Source: CAD feature listing. Evaluate the final solid. Frame: model axes, mm. A direction names the side the tool comes from. Give positions to 0.01 mm unless a question says otherwise; leave off trailing zeros. Order: outer loops, then holes, each group sorted by start corner. A loop starts at its lowest first (then second) coordinate and runs counter-clockwise, first axis right, second up.
from build123d import *

# Parameters (mm, degrees)
SKETCH1_R           = 6
BOSS_EXTRUDE1_DEPTH = 2
SKETCH2_R           = 3.5
SKETCH2_R_2         = 2.5
BOSS_EXTRUDE2_DEPTH = 3
SKETCH3_R           = 0.75
CUT_EXTRUDE1_DEPTH  = 2.5
CHAMFER1_SIZE       = 0.5
SKETCH5_R           = 1.25
CUT_EXTRUDE3_DEPTH  = 10.848857924


with BuildPart() as part:
    # Sketch1 → Boss-Extrude1 (new body)
    with BuildSketch(Plane.XY):
        Circle(SKETCH1_R)
    extrude(amount=BOSS_EXTRUDE1_DEPTH)

    # Sketch2 → Boss-Extrude2 (add)
    with BuildSketch(Plane(origin=(0, 0, 0), x_dir=(-1, 0, 0), z_dir=(0, 0, -1))):
        with Locations(Location((0, 0, 0), (0, 0, 180))):
            Circle(SKETCH2_R)
        Circle(SKETCH2_R_2, mode=Mode.SUBTRACT)
    extrude(amount=BOSS_EXTRUDE2_DEPTH)

    # Sketch3 → Cut-Extrude1 (cut)
    with BuildSketch(Plane.XY.offset(2)):
        with Locations((0, 5)):
            Circle(SKETCH3_R)
        with Locations((5.001, 0.001)):
            Circle(SKETCH3_R)
        with Locations((0.002, -5)):
            Circle(SKETCH3_R)
        with Locations((-4.999, -0.001)):
            Circle(SKETCH3_R)
    extrude(amount=-CUT_EXTRUDE1_DEPTH, mode=Mode.SUBTRACT)

    # Chamfer1
    # the kernel refuses this chamfer: 0.5 mm, written as the material it takes off along each edge
    with BuildSketch(Plane(origin=(0, 0, 0), x_dir=(1, 0, 0), z_dir=(0, -1, 0))) as chamfer1_piece_1:
        Polygon((6, CHAMFER1_SIZE), (6 - CHAMFER1_SIZE, 0), (6, 0), align=None)
    revolve(axis=Axis((0, 0, 0), (0, 0, 1)), mode=Mode.SUBTRACT)
    with BuildSketch(Plane(origin=(0, 0, 2), x_dir=(1, 0, 0), z_dir=(0, -1, 0))) as chamfer1_piece_2:
        Polygon((6, -CHAMFER1_SIZE), (6 - CHAMFER1_SIZE, 0), (6, 0), align=None)
    revolve(axis=Axis((0, 0, 2), (0, 0, 1)), mode=Mode.SUBTRACT)
    with BuildSketch(Plane(origin=(0, 0, -3), x_dir=(1, 0, 0), z_dir=(0, 1, 0))) as chamfer1_piece_3:
        Polygon((3.5, -CHAMFER1_SIZE), (3.5 - CHAMFER1_SIZE, 0), (3.5, 0), align=None)
    revolve(axis=Axis((0, 0, -3), (0, 0, -1)), mode=Mode.SUBTRACT)

    # Sketch5 → Cut-Extrude3 (cut, through all)
    with BuildSketch(Plane.XY.offset(2)):
        Circle(SKETCH5_R)
    extrude(amount=-CUT_EXTRUDE3_DEPTH, mode=Mode.SUBTRACT)


solid = part.part
1) Section query A-A on z = -0.75. Output: boundary loops of the cut face in (x, y), and give its area (3 significant figures).
Checks:
outline: circle Ø7 at (0, 0); hole circle Ø5 at (0, 0)
area: 18.8 mm2
2) Section query B-B on z = 1.05. Output: boundary loops of the cut face in (x, y), and give its area (3 significant figures).
Checks:
outline: circle Ø12 at (0, 0); hole circle Ø1.5 at (-5, 0); hole circle Ø2.5 at (0, 0); hole circle Ø1.5 at (0, -5); hole circle Ø1.5 at (0, 5); hole circle Ø1.5 at (5, 0)
area: 101 mm2
3) Ray query, L1, parallel to Y at x = 0, z = 1; L2, parallel to Y at x = -1.75, z = -2; L3, parallel to X at y = -2.25, z = -2.45. Return the intervals inside material, ascending.
Checks:
L1: y = -6 to -5.75, -4.25 to -1.25, 1.25 to 4.25, 5.75 to 6
L2: y = -3.03 to -1.79, 1.79 to 3.03
L3: x = -2.68 to -1.09, 1.09 to 2.68
4) Pull-direction query (X, two-part tool) for faces 3 (the face through (5.38, 1.69, 1.86)), 4 (the face through (1, 1, 0)), 5 (the face through (1, -1, 2)); classes: +X half, -X half, draft (parallel to the pull), parting line (faces both ways), or undercut.
Checks:
face 3: parting line
face 4: undercut
face 5: draft
5) Reachability of faces 1 (the face through (0, -4, 0)), 2 (the face through (-0.096, -4.256, 1.014)) from +Z, -Z, +X, -X, +Y, -Y: full face, straight path, thin tool, end or side. Return the list, or none.
Checks:
face 1: -Z
face 2: +Z, -Z
6) First-contact query: pin 1 Ø1 at (y, z) = (3, -2.5) entering from -X; pin 2 Ø1.5 at (y, z) = (-3.5, -1.5) entering from -X; pin 3 Ø2 at (x, y) = (-4.999, -0.001) entering from -Z. Flat tips, straight axial feed; report the tip coordinate or a pass-through.
Checks:
pin 1: stops at x = -2.45
pin 2: stops at x = -2.17
pin 3: stops at z = 0
